```python
from build123d import *

# Parameters (mm, degrees)
F0_R     = 9.09955
F1_DEPTH = 64.4906
F2_R     = 6.35
F3_DEPTH = 0.508


# Not quite as in the source:
# - a fillet or chamfer that OpenCascade refuses, or shapes differently, is made with other operations: its cross-section is extruded or revolved along the edge and cut away or added


with BuildPart() as f1:
    # F0 (on Front) → F1 (new body)
    with BuildSketch(Plane.XZ):
        Circle(F0_R)
    extrude(amount=-F1_DEPTH)

    # F2 (on face) → F3 (join)
    with BuildSketch(Plane.XZ):
        Circle(F2_R)
    extrude(amount=F3_DEPTH)

    # F4: fillet of radius 1.27 on 3 edges, made by hand

    # F4_s1 → F4_t2 (revolve, cut)
    with BuildSketch(Plane.XY):
        with BuildLine():
            ThreePointArc((9.09955, 63.2206), (8.7275756121, 64.1186256121), (7.82955, 64.4906))
            Line((7.82955, 64.4906), (9.09955, 64.4906))
            Line((9.09955, 64.4906), (9.09955, 63.2206))
        make_face()
    revolve(axis=Axis((0, 64.4906, 0), (0, -1, 0)), mode=Mode.SUBTRACT)

    # F4_s3 → F4_t4 (revolve, cut)
    with BuildSketch(Plane.XY):
        with BuildLine():
            ThreePointArc((9.09955, 1.27), (8.7275756121, 0.3719743879), (7.82955, 0))
            Line((7.82955, 0), (9.09955, 0))
            Line((9.09955, 0), (9.09955, 1.27))
        make_face()
    revolve(axis=Axis((0, 0, 0), (0, -1, 0)), mode=Mode.SUBTRACT)

    # F4_s5 → F4_t6 (revolve, cut)
    with BuildSketch(Plane.XY):
        with BuildLine():
            ThreePointArc((6.35, 0), (5.9019612663, -0.3739225326), (5.334, -0.508))
            Line((5.334, -0.508), (6.35, -0.508))
            Line((6.35, -0.508), (6.35, 0))
        make_face()
    revolve(axis=Axis((0, -0.508, 0), (0, -1, 0)), mode=Mode.SUBTRACT)


solid = f1.part
```
The listing builds one solid part. Answer for the finished solid, in the listing's coordinates (mm). A direction names the side the tool comes from. Round coordinates to 2 decimals unless told otherwise and drop trailing zeros. Loops run counter-clockwise (first coordinate to the right, second up) from the corner with the lowest first, then second, coordinate; pieces in that order, holes last. Notation, with made-up numbers: (68, 24) - (116, 24) arc R23 ccw to (116, 42) - close; hole circle Ø8 at (68.25, 67). An arc over 180 degrees is marked (long way). Use one line per item in the form item = value. Start each with the question number.
1. Given pin 1 Ø3 at (x, y) = (-4.5, 13) entering from -Z; pin 2 Ø1.5 at (y, z) = (53, 4) entering from -X; pin 3 Ø1 at (x, y) = (-3, 8) entering from -Z, each flat-ended and moving along its own axis, determine where each tip first touches the part or whether it passes through.
2. Consider line 1 (Y direction, x = -0.5, z = -7); line 2 (Y direction, x = -6, z = -0.75); line 3 (X direction, y = 40, z = 0.5). Determine where each line is inside the solid, lowest interval first. Write a range as [from, to].
3. The part is cut by section A-A on y = 53. Determine the outline of the cut face in (x, z).
4. A tool of negligible diameter and unlimited length cuts with its end or side. For faces 1 (the face through (0, 64.491, 0)), 2 (the face through (-1.2, 0, 6.4)), from which of +Z, -Z, +X, -X, +Y, -Y can it reach the whole face along a straight path? Write none if from no direction.
Geometry check:
q1.pin_1 = -8.59
q1.pin_2 = -8.5
q1.pin_3 = -8.75
q2.line_1 = [0, 64.49]
q2.line_2 = [-0.29, 64.49]
q2.line_3 = [-9.09, 9.09]
q3.outline = circle Ø18.2 at (0, 0)
q4.face_1 = +Z, -Z, +X, -X, +Y
q4.face_2 = -Y
